Check sheet for the drawn part. Datum: minimum x, y, z corner. Units: mm. Give positions to 0.01 mm unless a question says otherwise; leave off trailing zeros. Loops run counter-clockwise (first coordinate to the right, second up) from the corner with the lowest first, then second, coordinate; pieces in that order, holes last. Notation, with made-up numbers: (41, -33.5) - (79, -33.5) arc R16 ccw to (79, -14.5) - close; hole circle Ø1 at (5, 71). An arc over 180 degrees is marked (long way). One line per item, written item: value. Start each with the question number.
1. Sectioned sample at C-C (x = 2.4). Record the cut outline in (y, z), plus the area to 3 significant figures.
2. Sectioned sample at B-B (z = 30). Record the cut outline in (x, y), plus the area to 3 significant figures.
3. Scan lines: L1, parallel to Y at x = 2.1, z = 34.5; L2, parallel to Z at x = 4, y = 30; L3, parallel to Z at x = 1, y = 73. Record each from-to range of solid material in increasing order. Write a range as [from, to].
4. Sectioned sample at A-A (y = 70). Record the cut outline in (x, z), plus the area to 3 significant figures.
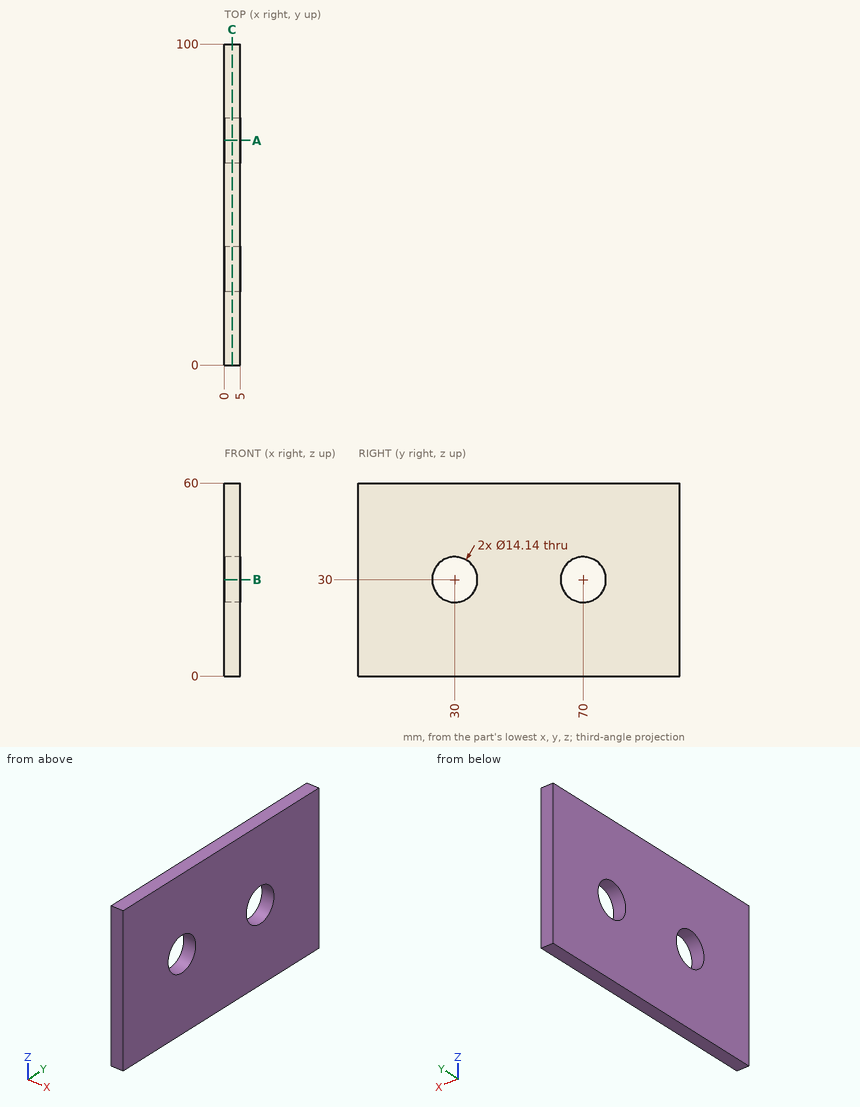
Results are:
1. outline: (0, 0) - (100, 0) - (100, 60) - (0, 60) - close; hole circle Ø14.14 at (30, 30); hole circle Ø14.14 at (70, 30)
1. area: 5,690 mm^2
2. outline: (0, 0) - (5, 0) - (5, 22.93) - (0, 22.93) - close; (0, 37.07) - (5, 37.07) - (5, 62.93) - (0, 62.93) - close; (0, 77.07) - (5, 77.07) - (5, 100) - (0, 100) - close
2. area: 359 mm^2
3. L1: y = [0, 24.55], [35.45, 64.55], [75.45, 100]
3. L2: z = [0, 22.93], [37.07, 60]
3. L3: z = [0, 23.6], [36.4, 60]
4. outline: (0, 0) - (5, 0) - (5, 22.93) - (0, 22.93) - close; (0, 37.07) - (5, 37.07) - (5, 60) - (0, 60) - close
4. area: 229 mm^2
